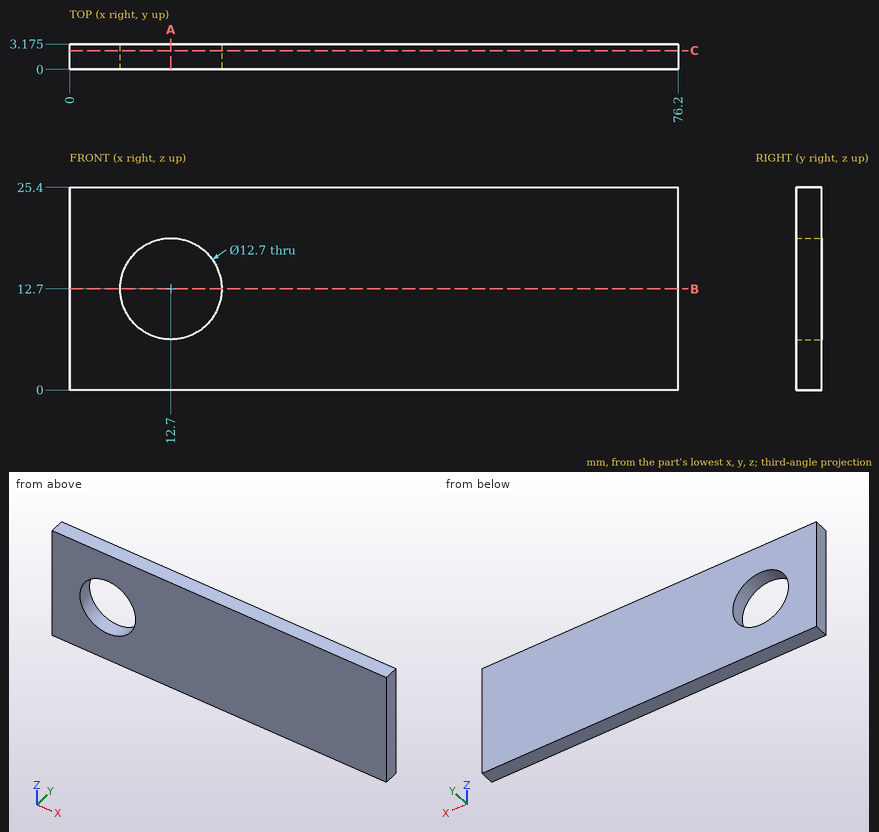
Geometry check sheet. Reference: drawing and pictorial views, mm from the part's lowest x, y, z. Coordinates: 2 decimals unless noted, no trailing zeros. Order: outer loops, then holes, each group sorted by start corner. A loop starts at its lowest first (then second) coordinate and runs counter-clockwise, first axis right, second up. Notation, with made-up numbers: (-38, 84) - (-7, 84) arc R28 cw to (-7, 119) - close; hole circle Ø6 at (1.25, 19). An arc over 180 degrees is marked (long way). Answer in a Markdown table with one row per item. Add a question column.
1) Cross-section at A-A, the plane x = 12.7. Record the cut outline in (y, z) (3 decimals), then the cut area to 3 significant figures.
2) Gauge pin test, flat end, axial feed: P1, Ø4, axis at x = 54.5, z = 5.5, coming from the -Y side. Record the tip position at first contact, or that the pin passes through.
3) Material ranges on line 1 along X through (y, z) = (2.45, 12.7); line 2 along Z through (x, y) = (12.7, 1.3); line 3 along Z through (x, y) = (11, 1.8), recorded low to high. Write a range as [from, to].
4) Cross-section at C-C, the plane y = 2.35. Record the cut outline in (x, z).
5) Cross-section at B-B, the plane z = 12.7. Record the cut outline in (x, y) (3 decimals).
Check result:
| question | item | result |
|---|---|---|
| 1 | outline | (0, 0) - (3.175, 0) - (3.175, 6.35) - (0, 6.35) - close; (0, 19.05) - (3.175, 19.05) - (3.175, 25.4) - (0, 25.4) - close |
| 1 | area | 40.3 mm² |
| 2 | P1 | stops at y = 0 |
| 3 | line 1 | x = [0, 6.35], [19.05, 76.2] |
| 3 | line 2 | z = [0, 6.35], [19.05, 25.4] |
| 3 | line 3 | z = [0, 6.58], [18.82, 25.4] |
| 4 | outline | (0, 0) - (76.2, 0) - (76.2, 25.4) - (0, 25.4) - close; hole circle Ø12.7 at (12.7, 12.7) |
| 5 | outline | (0, 0) - (6.35, 0) - (6.35, 3.175) - (0, 3.175) - close; (19.05, 0) - (76.2, 0) - (76.2, 3.175) - (19.05, 3.175) - close |
